The model under review builds one solid part; all positions refer to its coordinate system, in mm. A direction names the side the tool comes from. Round coordinates to 2 decimals unless told otherwise and drop trailing zeros. Write each loop counter-clockwise with the first axis right and the second up, starting at its lowest first coordinate (ties: lowest second). Pieces come first, ordered by that corner, then holes. Notation, with made-up numbers: (-19, 39) - (32, 39) arc R9 ccw to (32, 51) - close; hole circle Ø1 at (89.25, 9). An arc over 180 degrees is marked (long way). One line per question, with ' | ' between items. Start each with the question number.
Autodesk Inventor part; units mm, degrees
ref_plane "YZ Plane" through (0, 0, 0) normal (1, 0, 0) x (0, 1, 0)
ref_plane "XZ Plane" through (0, 0, 0) normal (0, 1, 0) x (-1, 0, 0)
ref_plane "XY Plane" through (0, 0, 0) normal (0, 0, 1) x (1, 0, 0)
sketch "Sketch1" plane through (0, 0, 0) normal (0, 1, 0) x (-1, 0, 0)
  circle A0 centre (0, 0) radius 2.0828
  dimension "d4" = 4.1656
extrude "Body" add sketch "Sketch1" along normal blind 9.525
sketch "Sketch2" plane through (0, 0, 0) normal (1, 0, 0) x (0, 1, 0)
  line L0 (9.525, -2.0828) -> (9.525, 2.0828)
  line L1 (9.525, 0) -> (9.525, -3.9624)
  line L2 (9.525, -3.9624) -> (9.906, -3.9624)
  arc A0 (9.906, -3.9624) -> (11.7348, -2.0828) centre (7.7138, 0) ccw
  line L3 (11.7348, -2.0828) -> (11.7348, -1.6764)
  line L4 (11.7348, -1.6764) -> (10.2385, -1.6764)
  line L5 (10.2385, -1.6764) -> (9.6266, 0)
  line L6 (9.6266, 0) -> (9.525, 0)
  point P0 (0, 0)
  dimension "d5" = 3.9624
  dimension "d6" = 0.381
  dimension "d13" = 0.1016
  dimension "d14" = 2.0828
  dimension "d15" = 2.2098
  dimension "d16" = 0
  dimension "d17" = 1.6764
  dimension "d57" = 20.053
revolve "Head" add sketch "Sketch2" angle 360 about axis through (0, 9.6266, 0) along (0, -1, 0)
sketch "Sketch3" plane through (0, 11.7348, 0) normal (0, 1, 0) x (1, 0, 0)
  circle A0 centre (0, 0) radius 1.6764
  line L0 (0.7302, -1.2648) -> (-0.7303, -1.2648) construction
  line L1 (-0.7303, -1.2648) -> (-1.4605, 0) construction
  line L2 (-1.4605, 0) -> (-0.7303, 1.2648) construction
  line L3 (-0.7303, 1.2648) -> (0.7302, 1.2648) construction
  line L4 (0.7302, 1.2648) -> (1.4605, 0) construction
  line L5 (1.4605, 0) -> (0.7302, -1.2648) construction
  circle A1 centre (-0.7303, -1.2648) radius 0.2159
  circle A2 centre (-1.4605, 0) radius 0.2159
  circle A3 centre (-0.7303, 1.2648) radius 0.2159
  circle A4 centre (0.7302, 1.2648) radius 0.2159
  circle A5 centre (1.4605, 0) radius 0.2159
  circle A6 centre (0.7302, -1.2648) radius 0.2159
  circle A7 centre (0, -2.0701) radius 0.8712
  circle A8 centre (0, 2.0701) radius 0.8712
  circle A9 centre (1.7928, -1.0351) radius 0.8712
  circle A10 centre (-1.7928, 1.035) radius 0.8712
  circle A11 centre (1.7928, 1.035) radius 0.8712
  circle A12 centre (-1.7928, -1.0351) radius 0.8712
  circle A13 centre (0, 0) radius 1.8188
  point P0 (0, 0)
  point P1 (0, 0)
  point P2 (0.9413, 1.2192)
  point P3 (1.5265, 0.2056)
  point P4 (1.5265, -0.2056)
  point P5 (0.9413, -1.2192)
  point P6 (0.5852, -1.4248)
  point P7 (-0.5852, -1.4248)
  point P8 (-0.9413, -1.2192)
  point P9 (-1.5265, -0.2056)
  point P10 (-1.5265, 0.2056)
  point P11 (-0.9413, 1.2192)
  point P12 (-0.5852, 1.4248)
  point P13 (0.5852, 1.4248)
  dimension "d58" = 2.921
  dimension "d59" = 4.1402
  dimension "d62" = 120
extrude "Hex" add sketch "Sketch3" against normal blind 1.778 contours A5 A11 A0 | A0 A11 A13 A9 | A0 A9 A5 | A11 A0 | A0 A11 A13 | A9 A13 A0 | A0 A9 | A11 A4 A0 | A0 A8 A13 A11 | A9 A13 A7 A0 | A0 A6 A9 | A4 A8 A0 | A0 A7 A6 | A8 A0 | A7 A0 | A0 A8 A13 | A7 A13 A0 | A3 A0 A8 | A7 A0 A1 | A0 A10 A13 A8 | A7 A13 A12 A0 | A3 A10 A0 | A0 A12 A1 | A10 A0 A13 | A13 A12 A0 | A10 A0 | A0 A12 | A10 A0 A12 A13 | A10 A2 A0 | A0 A2 A12
sketch "Sketch4" plane through (0, 0, 0) normal (0, 0, 1) x (1, 0, 0)
  line L0 (-0.7364, 10.7948) -> (-1.6764, 11.7348)
  line L1 (0, 11.7348) -> (-0.7364, 10.7948)
  line L2 (0, -1.712) -> (0, 10.2718)
  line L3 (-1.5265, 11.7348) -> (-1.5265, 10.1888)
  line L4 (-1.5265, 11.7348) -> (-1.5265, 11.7348)
  line L5 (-1.5265, 11.7348) -> (-1.5265, 10.1888)
  line L6 (-1.6764, 11.7348) -> (-1.5265, 11.7348)
  line L7 (-1.6764, 11.7348) -> (0, 11.7348)
  point P0 (0, 0)
  point P1 (-1.6764, 10.2385)
  dimension "d29" = 1.6764
revolve "Head Chamfer" cut sketch "Sketch4" angle 360 about axis through (0, -10, 0) along (0, 1, 0)
sketch "Sketch5" plane through (0, 0, 0) normal (1, 0, 0) x (0, 1, 0)
  line L0 (0, -2.0828) -> (9.525, -2.0828)
  line L1 (9.525, 3.9624) -> (9.525, -3.9624)
  line L2 (9.525, -2.0828) -> (9.525, 2.0828)
  line L3 (0.0745, -2.0828) -> (-0.2261, -2.6035)
  line L4 (-0.2261, -2.6035) -> (-0.3253, -2.6035)
  line L5 (-0.3253, -2.6035) -> (-0.626, -2.0828)
  line L6 (0.0686, -2.6035) -> (-0.7252, -2.6035) construction
  line L7 (-0.626, -2.0828) -> (0.0745, -2.0828)
  line L8 (0, -2.0828) -> (9.525, -2.0828)
  point P0 (0, 0)
  dimension "d31" = 30
  dimension "d32" = 60
  dimension "a" = 0.0992
  dimension "d46" = 0.7937
  dimension "d54" = 0.0686
  dimension "d55" = 0.5207
  dimension "d56" = 0.0992
feature "Thread" [suppressed]
sketch "Sketch6" plane through (0, 0, 0) normal (0, 0, 1) x (1, 0, 0)
  line L0 (0, 0) -> (-1.4859, 0)
  line L1 (2.0828, 0) -> (-2.0828, 0)
  line L2 (-1.4859, 0) -> (-2.4948, 1.0089)
  line L3 (-2.4948, 1.0089) -> (-2.9651, -1.2188)
  line L4 (-2.9651, -1.2188) -> (-1.4859, -1.2188)
  line L5 (-2.0828, 0) -> (-2.0828, 9.525)
  line L6 (-1.4859, -1.2188) -> (-1.4859, 0)
  line L7 (0, -2.7326) -> (0, 7.8638)
  point P0 (-2.0828, 0.5969)
  dimension "d49" = 1.4859
  dimension "d50" = 135
revolve "Tapered End" cut sketch "Sketch6" angle 360 about axis through (0, -10, 0) along (0, 1, 0)
equation "\"d56\" = a"
properties part number "Screw 8-32 Steel 2.500" material "VEX Steel"
1. Machinability: for faces 4 (the face through (-2, 9.525, -2)), 5 (the face through (-3.93, 9.72, 0.52)), 6 (the face through (-1.043, 10.672, -0.592)), which of the approach directions +Z, -Z, +X, -X, +Y, -Y give a long, thin tool a straight path to every point of the face, cutting with its end or side? Answer none if there is none.
2. The part is to be moulded in two halves that separate along Z. For faces 1 (the face through (0, 0, 0)), 2 (the face through (-1.987, 4.998, -0.626)), 3 (the face through (0.102, 9.665, 0.023)), say which applies: pulls with the +Z half, pulls with the -Z half, needs draft (parallel to the pull), parting line crosses it, or undercut.
3. Add section A-A, the plane y = 7.25. Write out the cut boundary in (x, z).
4. Wall thickness on line 1 along X through (y, z) = (4.5, 0); line 2 along Y through (x, z) = (-0.5, -3.5) (3 decimals); line 3 along Z through (x, y) = (0.75, 3.5): over which ranges is each line inside the solid? List them lowest first. Write a range as [from, to].
5. Clearance check with flat-ended pins moving along their axes: P1, Ø1.5, axis at x = 0, y = 4, coming from the +Z side; P2, Ø2, axis at y = 4, z = 0.5, coming from the +X side; P3, Ø2, axis at x = -1.5, y = 2, coming from the -Z side. State where each tip first meets the part, or that it passes through.
Geometry check:
1) face 4: -Y | face 5: +Y, -Y | face 6: +Y
2) face 1: needs draft | face 2: parting line crosses it | face 3: undercut
3) outline: circle Ø4.17 at (0, 0)
4) line 1: x = [-2.08, 2.08] | line 2: y = [9.525, 10.543] | line 3: z = [-1.94, 1.94]
5) P1: stops at z = 2.08 | P2: stops at x = 2.08 | P3: stops at z = -2.02
